Part model, mm, in its own coordinate system. Face numbers are marked on the shaded views. A direction names the side the tool comes from. Give positions to 0.01 mm unless a question says otherwise; leave off trailing zeros. Loops run counter-clockwise (first coordinate to the right, second up) from the corner with the lowest first, then second, coordinate; pieces in that order, holes last. Notation, with made-up numbers: M 14.25,72.5 L 40.25,72.5 A16 cw 40.25,91.5 Z; hole C 43.25,21 d7. An arc over 180 degrees is marked long. Put each result on its own line as item: value. Start each with the question number.
```python
from build123d import *

# Parameters (mm, degrees)
BOSS_EXTRUDE1_DEPTH  = 1.905
BOSS_EXTRUDE3_DEPTH  = 3.429
BOSS_EXTRUDE2_DEPTH  = 3.81
LPATTERN1_COUNT      = 10
LPATTERN1_PITCH      = 2.54
MIRROR1_COPY_1_DEPTH = 3.81
MIRROR1_COPY_2_DEPTH = 3.81
MIRROR1_COPY_3_DEPTH = 3.81
MIRROR1_COPY_4_DEPTH = 3.81
MIRROR1_COPY_5_DEPTH = 3.81
MIRROR1_COPY_6_DEPTH = 3.81
MIRROR1_COPY_7_DEPTH = 3.81
MIRROR1_COPY_8_DEPTH = 3.81
MIRROR1_COPY_9_DEPTH = 3.81
BOSS_EXTRUDE4_DEPTH  = 1.27
SKETCH5_R            = 2.54
CUT_EXTRUDE1_DEPTH   = 31.555296323
SKETCH6_R            = 3.81
SKETCH6_R_2          = 2.54
BOSS_EXTRUDE5_DEPTH  = 7.62


with BuildPart() as part:
    # Sketch1 → Boss-Extrude1 (new, symmetric)
    with BuildSketch(Plane.XY):
        with BuildLine():
            Line((-3.754374137, -0.648671595), (-8.255, 25.4))
            Line((-8.255, 25.4), (8.255, 25.4))
            Line((8.255, 25.4), (3.754374137, -0.648671595))
            ThreePointArc((3.754374137, -0.648671595), (0, -3.81), (-3.754374137, -0.648671595))
        make_face()
    extrude(amount=BOSS_EXTRUDE1_DEPTH, both=True)

    # Sketch3 → Boss-Extrude3 (add)
    with BuildSketch(Plane(origin=(0, 0, -1.905), x_dir=(-1, 0, 0), z_dir=(0, 0, -1))):
        with BuildLine():
            Line((6.966183323, 25.4), (-6.966183323, 25.4))
            Line((-6.966183323, 25.4), (-2.502916091, -0.43244773))
            ThreePointArc((-2.502916091, -0.43244773), (0, -2.54), (2.502916091, -0.43244773))
            Line((2.502916091, -0.43244773), (6.966183323, 25.4))
        make_face()
    extrude(amount=BOSS_EXTRUDE3_DEPTH)

    # Sketch2 → Boss-Extrude2 (add)
    with BuildSketch(Plane.XY.offset(1.905)):
        Polygon((-3.754374137, -0.648671595), (-6.726821867, 1.4153895), (-4.186821867, 1.854244497), align=None)
    boss_extrude2 = extrude(amount=-BOSS_EXTRUDE2_DEPTH)

    # LPattern1: Boss-Extrude2 ×10
    with Locations(*[Vector(-0.17025501170659457, 0.9854000360202892, 0) * (i * LPATTERN1_PITCH) for i in range(1, LPATTERN1_COUNT)]):
        add(boss_extrude2)

    # Mirror1: Boss-Extrude2 across plane
    add(boss_extrude2.mirror(Plane(origin=(0, 0, 0), x_dir=(0, 0, 1), z_dir=(1, 0, 0))))

    # Mirror1 copy 1 sketch → Mirror1 copy 1 (add)
    with BuildSketch(Plane(origin=(0.43244773, 2.502916091, 1.905), x_dir=(-1, 0, 0), z_dir=(0, 0, 1))):
        Polygon((-3.754374137, 0.648671595), (-6.726821867, -1.4153895), (-4.186821867, -1.854244497), align=None)
    extrude(amount=-MIRROR1_COPY_1_DEPTH)

    # Mirror1 copy 2 sketch → Mirror1 copy 2 (add)
    with BuildSketch(Plane(origin=(0.864895459, 5.005832183, 1.905), x_dir=(-1, 0, 0), z_dir=(0, 0, 1))):
        Polygon((-3.754374137, 0.648671595), (-6.726821867, -1.4153895), (-4.186821867, -1.854244497), align=None)
    extrude(amount=-MIRROR1_COPY_2_DEPTH)

    # Mirror1 copy 3 sketch → Mirror1 copy 3 (add)
    with BuildSketch(Plane(origin=(1.297343189, 7.508748274, 1.905), x_dir=(-1, 0, 0), z_dir=(0, 0, 1))):
        Polygon((-3.754374137, 0.648671595), (-6.726821867, -1.4153895), (-4.186821867, -1.854244497), align=None)
    extrude(amount=-MIRROR1_COPY_3_DEPTH)

    # Mirror1 copy 4 sketch → Mirror1 copy 4 (add)
    with BuildSketch(Plane(origin=(1.729790919, 10.011664366, 1.905), x_dir=(-1, 0, 0), z_dir=(0, 0, 1))):
        Polygon((-3.754374137, 0.648671595), (-6.726821867, -1.4153895), (-4.186821867, -1.854244497), align=None)
    extrude(amount=-MIRROR1_COPY_4_DEPTH)

    # Mirror1 copy 5 sketch → Mirror1 copy 5 (add)
    with BuildSketch(Plane(origin=(2.162238649, 12.514580457, 1.905), x_dir=(-1, 0, 0), z_dir=(0, 0, 1))):
        Polygon((-3.754374137, 0.648671595), (-6.726821867, -1.4153895), (-4.186821867, -1.854244497), align=None)
    extrude(amount=-MIRROR1_COPY_5_DEPTH)

    # Mirror1 copy 6 sketch → Mirror1 copy 6 (add)
    with BuildSketch(Plane(origin=(2.594686378, 15.017496549, 1.905), x_dir=(-1, 0, 0), z_dir=(0, 0, 1))):
        Polygon((-3.754374137, 0.648671595), (-6.726821867, -1.4153895), (-4.186821867, -1.854244497), align=None)
    extrude(amount=-MIRROR1_COPY_6_DEPTH)

    # Mirror1 copy 7 sketch → Mirror1 copy 7 (add)
    with BuildSketch(Plane(origin=(3.027134108, 17.52041264, 1.905), x_dir=(-1, 0, 0), z_dir=(0, 0, 1))):
        Polygon((-3.754374137, 0.648671595), (-6.726821867, -1.4153895), (-4.186821867, -1.854244497), align=None)
    extrude(amount=-MIRROR1_COPY_7_DEPTH)

    # Mirror1 copy 8 sketch → Mirror1 copy 8 (add)
    with BuildSketch(Plane(origin=(3.459581838, 20.023328732, 1.905), x_dir=(-1, 0, 0), z_dir=(0, 0, 1))):
        Polygon((-3.754374137, 0.648671595), (-6.726821867, -1.4153895), (-4.186821867, -1.854244497), align=None)
    extrude(amount=-MIRROR1_COPY_8_DEPTH)

    # Mirror1 copy 9 sketch → Mirror1 copy 9 (add)
    with BuildSketch(Plane(origin=(3.892029568, 22.526244823, 1.905), x_dir=(-1, 0, 0), z_dir=(0, 0, 1))):
        Polygon((-3.754374137, 0.648671595), (-6.726821867, -1.4153895), (-4.186821867, -1.854244497), align=None)
    extrude(amount=-MIRROR1_COPY_9_DEPTH)

    # Sketch4 → Boss-Extrude4 (add)
    with BuildSketch(Plane(origin=(0, 0, -5.334), x_dir=(-1, 0, 0), z_dir=(0, 0, -1))):
        with BuildLine():
            Line((-14.699083385, 25.4), (14.699083385, 25.4))
            Line((14.699083385, 25.4), (14.474931597, 24.102656811))
            Line((14.474931597, 24.102656811), (10.011664366, -1.729790919))
            ThreePointArc((10.011664366, -1.729790919), (0, -10.16), (-10.011664366, -1.729790919))
            Line((-10.011664366, -1.729790919), (-14.474931597, 24.102656811))
            Line((-14.474931597, 24.102656811), (-14.699083385, 25.4))
        make_face()
    extrude(amount=BOSS_EXTRUDE4_DEPTH)

    # Sketch5 → Cut-Extrude1 (cut, through all)
    with BuildSketch(Plane.XY.offset(1.905)):
        Circle(SKETCH5_R)
    extrude(amount=-CUT_EXTRUDE1_DEPTH, mode=Mode.SUBTRACT)

    # Sketch6 → Boss-Extrude5 (add)
    with BuildSketch(Plane.XY.offset(1.905)):
        Circle(SKETCH6_R)
        Circle(SKETCH6_R_2, mode=Mode.SUBTRACT)
    extrude(amount=-BOSS_EXTRUDE5_DEPTH)


solid = part.part
```
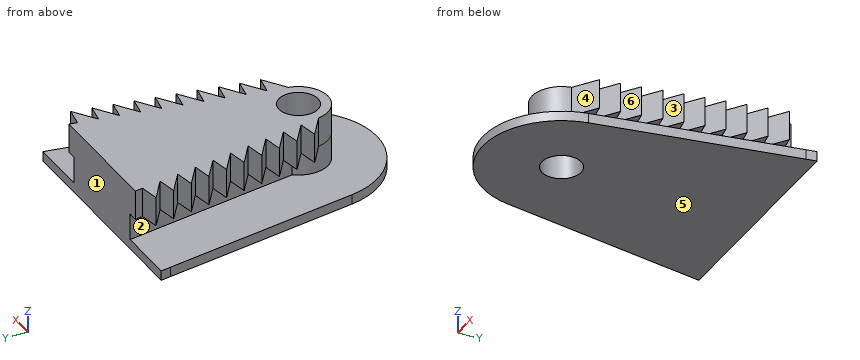
1) Band-saw the part on C-C on z = -3.5. Give the cut face in (x, y).
2) Pin check, flat tips, straight feed: pin 1 Ø3 at (y, z) = (-5.5, -4.5) entering from +X; pin 2 Ø1 at (y, z) = (1, -1.5) entering from +X. Stop position of each tip, or through.
3) Which spindle directions (+Z, -Z, +X, -X, +Y, -Y) get a long thin tool onto all of the face, cutting with end or side? Do the marked faces 1, 2 and 3. Say none if no direction does.
4) Band-saw the part on D-D on y = 18. Give the cut face in (x, z) (3 decimals), then the cut area to 3 significant figures.
5) Band-saw the part on A-A on x = 0. Give the cut face in (y, z) (3 decimals).
6) Band-saw the part on B-B on y = 0.5. Give the cut face in (x, z) (3 decimals).
7) Wall check: L1, parallel to Y at x = 0, z = -4.75; L2, parallel to Y at x = 5.75, z = 0; L3, parallel to Z at x = 4.75, y = 3.5 (3 decimals). Give the ranges that are in metal, low to high.
8) Mould opens along Y. For the marked faces 4, 5 and 6 say: +Y half, -Y half, draft (parallel to the pull), parting line (faces both ways), or undercut.
Evaluation:
1. outline: M -6.97,25.4 L -2.99,2.37 A3.81 ccw long 2.99,2.37 L 6.97,25.4 Z; hole C 0,0 d5.08
2. pin 1: x = 9.23
2. pin 2: x = 6.73
3. face 1: +Z, -Z, +X, -X, +Y
3. face 2: -X
3. face 3: +Z, +X
4. outline: M -13.421,-6.604 L 13.421,-6.604 L 13.421,-5.334 L 5.688,-5.334 L 5.688,-1.905 L 8.406,-1.905 L 8.406,1.905 L -8.406,1.905 L -8.406,-1.905 L -5.688,-1.905 L -5.688,-5.334 L -13.421,-5.334 Z
4. area: 137 mm2
5. outline: M -10.16,-6.604 L -2.54,-6.604 L -2.54,1.905 L -3.81,1.905 L -3.81,-5.334 L -10.16,-5.334 Z; M 2.54,-6.604 L 25.4,-6.604 L 25.4,1.905 L 2.54,1.905 Z
6. outline: M -10.397,-6.604 L -2.49,-6.604 L -2.49,1.905 L -5.409,1.905 L -5.409,-1.905 L -3.777,-1.905 L -3.777,-5.334 L -10.397,-5.334 Z; M 2.49,-6.604 L 10.397,-6.604 L 10.397,-5.334 L 3.777,-5.334 L 3.777,-1.905 L 5.409,-1.905 L 5.409,1.905 L 2.49,1.905 Z
7. L1: -3.81 to -2.54, 2.54 to 25.4
7. L2: 0.74 to 1.58, 2.94 to 4.16, 5.14 to 6.74, 7.34 to 9.32, 9.55 to 25.4
7. L3: -6.604 to -5.334, -1.905 to 1.905
8. face 4: -Y half
8. face 5: draft
8. face 6: undercut
